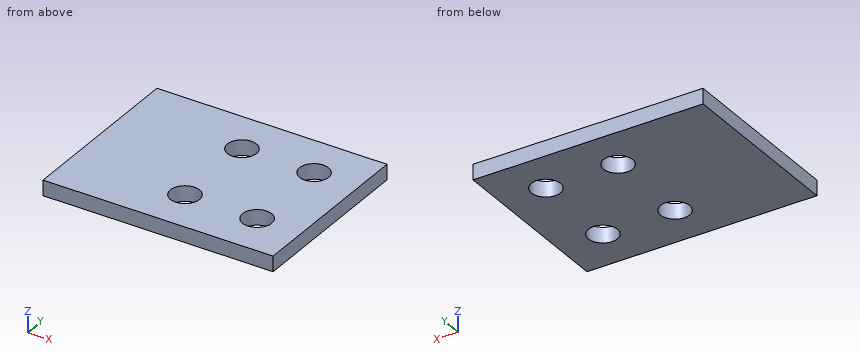
Solid Edge part; units mm, degrees
sketch "Sketch1" plane through (0, 0, 0) normal (0, 0, 1) x (1, 0, 0)
  line L0 (75, -58) -> (75, 58)
  line L1 (75, 58) -> (-75, 58)
  line L2 (-75, 58) -> (-75, -58)
  line L3 (-75, -58) -> (75, -58)
extrude "Protrusion1" add sketch "Sketch1" against normal blind 10
sketch "Sketch2" plane through (0, 0, 0) normal (0, 0, 1) x (1, 0, 0)
  circle A0 centre (46, 29) radius 9.5
extrude "ExtrudedCutout_1" cut sketch "Sketch2" against normal blind 10
pattern_linear "Pattern1" count 2 spacing 47 along (-1, 0, 0) count 2 spacing 58 along (0, -1, 0) of "ExtrudedCutout_1"
Check sheet for the modelled part. Datum: model origin and axes. Units: mm. Round coordinates to 2 decimals unless told otherwise and drop trailing zeros. Write each loop counter-clockwise with the first axis right and the second up, starting at its lowest first coordinate (ties: lowest second). Pieces come first, ordered by that corner, then holes. Notation, with made-up numbers: (-7, -37) -> (43, -37) arc R19 ccw to (43, -10) -> close; hole circle Ø5 at (77, 76.25). An arc over 180 degrees is marked (long way). Answer as CSV lines item,"result". Start each with the question number.
1) Go/stop test with flat-tipped pins: P1, Ø11.5, axis at x = -1, y = 29, coming from the -Z side; P2, Ø1.5, axis at x = 56.5, y = -17, coming from the +Z side. Record where each tip stops, or that it passes through.
2) Material ranges on line 1 (Y direction, x = -1, z = -2.5); line 2 (X direction, y = -24.5, z = -8.75); line 3 (X direction, y = 32.5, z = -6.5), recorded low to high. Write a range as from..to.
3) Section check B-B on x = 46. Enter the section's corners in (y, z).
4) Section check C-C on z = -4.75. Enter the section's corners in (x, y).
5) Section check A-A on y = 29. Enter the section's corners in (x, z).
Found:
1,P1,"passes through"
1,P2,"stops at z = 0"
2,line 1,"y = -58..-38.5, -19.5..19.5, 38.5..58"
2,line 2,"x = -75..-9.37, 7.37..37.63, 54.37..75"
2,line 3,"x = -75..-9.83, 7.83..37.17, 54.83..75"
3,outline,"(-58, -10) -> (-38.5, -10) -> (-38.5, 0) -> (-58, 0) -> close; (-19.5, -10) -> (19.5, -10) -> (19.5, 0) -> (-19.5, 0) -> close; (38.5, -10) -> (58, -10) -> (58, 0) -> (38.5, 0) -> close"
4,outline,"(-75, -58) -> (75, -58) -> (75, 58) -> (-75, 58) -> close; hole circle Ø19 at (-1, -29); hole circle Ø19 at (-1, 29); hole circle Ø19 at (46, -29); hole circle Ø19 at (46, 29)"
5,outline,"(-75, -10) -> (-10.5, -10) -> (-10.5, 0) -> (-75, 0) -> close; (8.5, -10) -> (36.5, -10) -> (36.5, 0) -> (8.5, 0) -> close; (55.5, -10) -> (75, -10) -> (75, 0) -> (55.5, 0) -> close"
